Check sheet for the modelled part. Datum: model origin and axes. Units: mm. Face numbers are marked on the shaded views. A direction names the side the tool comes from. Give positions to 0.01 mm unless a question says otherwise; leave off trailing zeros. Write each loop counter-clockwise with the first axis right and the second up, starting at its lowest first coordinate (ties: lowest second). Pieces come first, ordered by that corner, then holes.
from build123d import *

# Parameters (mm, degrees)
SKETCH_1_R      = 1
SKETCH_1_R_2    = 1.5
EXTRUDE_1_DEPTH = 10
SKETCH_3_W      = 58.885714286
SKETCH_3_H      = 63.4
SKETCH_3_W_2    = 54.885714286
SKETCH_3_H_2    = 59.4
EXTRUDE_2_DEPTH = 1.4
FILLET_1_R      = 3


with BuildPart() as part:
    # Эскиз1 → Бобышка-Вытянуть1 (new body)
    with BuildSketch(Plane(origin=(0, 0, 0), x_dir=(1, 0, 0), z_dir=(0, 1, 0))):
        with BuildLine():
            Line((-4, 4), (16, 4))
            ThreePointArc((16, 4), (20, 8), (24, 4))
            Line((24, 4), (62.885714286, 4))
            Line((62.885714286, 4), (62.885714286, 1.233529339))
            ThreePointArc((62.885714286, 1.233529339), (65.2, -2.7), (62.885714286, -6.633529339))
            Line((62.885714286, -6.633529339), (62.885714286, -56.766470661))
            ThreePointArc((62.885714286, -56.766470661), (65.2, -60.7), (62.885714286, -64.633529339))
            Line((62.885714286, -64.633529339), (62.885714286, -67.4))
            Line((62.885714286, -67.4), (24, -67.4))
            ThreePointArc((24, -67.4), (20, -71.4), (16, -67.4))
            Line((16, -67.4), (-4, -67.4))
            Line((-4, -67.4), (-4, -64.866533331))
            ThreePointArc((-4, -64.866533331), (-6.8, -60.7), (-4, -56.533466669))
            Line((-4, -56.533466669), (-4, -6.866533331))
            ThreePointArc((-4, -6.866533331), (-6.8, -2.7), (-4, 1.466533331))
            Line((-4, 1.466533331), (-4, 4))
        make_face()
        with Locations(Location((-2.3, -2.7, 0), (0, 0, 270))):
            Circle(SKETCH_1_R, mode=Mode.SUBTRACT)
        with Locations(Location((60.7, -2.7, 0), (0, 0, 270))):
            Circle(SKETCH_1_R, mode=Mode.SUBTRACT)
        with Locations(Location((60.7, -60.7, 0), (0, 0, 270))):
            Circle(SKETCH_1_R, mode=Mode.SUBTRACT)
        with Locations(Location((-2.3, -60.7, 0), (0, 0, 270))):
            Circle(SKETCH_1_R, mode=Mode.SUBTRACT)
        with Locations(Location((20, -67.4, 0), (0, 0, 270))):
            Circle(SKETCH_1_R_2, mode=Mode.SUBTRACT)
        with Locations(Location((20, 4, 0), (0, 0, 270))):
            Circle(SKETCH_1_R_2, mode=Mode.SUBTRACT)
        with BuildLine():
            Line((1.5, 0), (57.385714286, 0))
            ThreePointArc((57.385714286, 0), (58.446374457, -0.439339828), (58.885714286, -1.5))
            Line((58.885714286, -1.5), (58.885714286, -61.9))
            ThreePointArc((58.885714286, -61.9), (58.446374457, -62.960660172), (57.385714286, -63.4))
            Line((57.385714286, -63.4), (1.5, -63.4))
            ThreePointArc((1.5, -63.4), (0.439339828, -62.960660172), (0, -61.9))
            Line((0, -61.9), (0, -1.5))
            ThreePointArc((0, -1.5), (0.439339828, -0.439339828), (1.5, 0))
        make_face(mode=Mode.SUBTRACT)
    extrude(amount=EXTRUDE_1_DEPTH)

    # Эскиз3 → Бобышка-Вытянуть2 (add)
    with BuildSketch(Plane.XZ):
        with Locations((29.442857143, 31.7)):
            Rectangle(SKETCH_3_W, SKETCH_3_H)
        with Locations((29.442857143, 31.7)):
            Rectangle(SKETCH_3_W_2, SKETCH_3_H_2, mode=Mode.SUBTRACT)
    extrude(amount=-EXTRUDE_2_DEPTH)

    # Скругление1
    # the kernel refuses this fillet: 3 mm, written as the material it takes off along each edge
    with BuildSketch(Plane(origin=(62.885714286, -7.477242159, 67.4), x_dir=(-1, 0, 0), z_dir=(0, 1, 0))) as fillet_1_piece_1:
        with BuildLine():
            CenterArc((2.990896863, -3), FILLET_1_R, 90, 85.535401485)
            Line((0, -2.766470661), (-0.059817937, -2.761800074))
            ThreePointArc((-0.059817937, -2.761800074), (-0.06, -1.38323533), (-0.06, 0))
            Line((-0.06, 0), (0, 0.06))
            Line((0, 0.06), (2.990896863, 0.06))
            Line((2.990896863, 0.06), (2.990896863, 0))
        make_face()
    extrude(amount=24.954484317, mode=Mode.SUBTRACT)
    with BuildSketch(Plane(origin=(-4, -7.408756074, 67.4), x_dir=(0, 0, -1), z_dir=(0, 1, 0))) as fillet_1_piece_2:
        with BuildLine():
            CenterArc((3, -2.96350243), FILLET_1_R, 98.946440174, 81.053559826)
            Line((0, -2.96350243), (-0.06, -2.96350243))
            Line((-0.06, -2.96350243), (-0.06, 0))
            Line((-0.06, 0), (0, 0.06))
            ThreePointArc((0, 0.06), (1.266733334, 0.06), (2.524136002, 0.059270049))
            Line((2.524136002, 0.059270049), (2.533466669, 0))
        make_face()
    extrude(amount=24.817512149, mode=Mode.SUBTRACT)
    with BuildSketch(Plane(origin=(62.885714286, -7.477242159, -4), x_dir=(-1, 0, 0), z_dir=(0, 1, 0))) as fillet_1_piece_3:
        with BuildLine():
            CenterArc((2.990896863, 3), FILLET_1_R, 184.464598515, 85.535401485)
            Line((0, 2.766470661), (-0.059817937, 2.761800074))
            ThreePointArc((-0.059817937, 2.761800074), (-0.06, 1.38323533), (-0.06, 0))
            Line((-0.06, 0), (0, -0.06))
            Line((0, -0.06), (2.990896863, -0.06))
            Line((2.990896863, -0.06), (2.990896863, 0))
        make_face()
    extrude(amount=24.954484317, mode=Mode.SUBTRACT)
    with BuildSketch(Plane(origin=(-4, -7.408756074, -4), x_dir=(0, 0, 1), z_dir=(0, 1, 0))) as fillet_1_piece_4:
        with BuildLine():
            CenterArc((3, 2.96350243), FILLET_1_R, 180, 81.053559826)
            Line((0, 2.96350243), (-0.06, 2.96350243))
            Line((-0.06, 2.96350243), (-0.06, 0))
            Line((-0.06, 0), (0, -0.06))
            ThreePointArc((0, -0.06), (1.266733334, -0.06), (2.524136002, -0.059270049))
            Line((2.524136002, -0.059270049), (2.533466669, 0))
        make_face()
    extrude(amount=24.817512149, mode=Mode.SUBTRACT)


solid = part.part
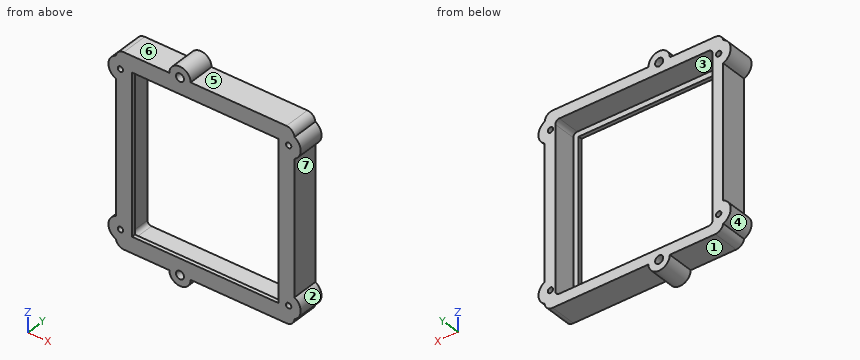
1) Draft check along X on the marked faces 1, 2, 3 and 4. Enter one of: +X half, -X half, draft (parallel to the pull), parting line (faces both ways), or undercut.
2) Sectioned sample at B-B on z = 14.5. Record the boundary of the cut face in (x, y), then the cut area to 3 significant figures.
3) Sectioned sample at A-A on x = 56. Record the boundary of the cut face in (y, z).
4) Sectioned sample at C-C on y = 5.25. Give the number of separate pieces and of enclosed holes in the cut face, then the cut area to 3 significant figures.
5) Scan lines: L1, parallel to X at y = 5, z = 60.7; L2, parallel to Z at x = 35, y = 8; L3, parallel to X at y = 5, z = 20.5. Record each from-to range of solid material in increasing order.
6) Gauge pin test, flat ends, axial feed: pin 1 (5 mm diameter, centred on x = 48, y = 3.5, fed in from +Z); pin 2 (1.5 mm diameter, centred on x = 3.5, y = 2, fed in from -Z); pin 3 (4.5 mm diameter, centred on x = 24, y = 7, fed in from +Z). Record the tip position at first contact, or that the pin passes through.
7) Sectioned sample at D-D on x = 20. Record the boundary of the cut face in (y, z).
8) Access from +Z, -Z, +X, -X, +Y, -Y to the whole of each face (thin tool, end or side, straight path). Record for the marked faces 5, 6 and 7.
Answers below:
1. face 1: draft
1. face 2: +X half
1. face 3: undercut
1. face 4: -X half
2. outline: (-4, 0) - (2, 0) - (2, 1.4) - (0, 1.4) - (0, 10) - (-4, 10) - close; (56.89, 0) - (62.89, 0) - (62.89, 10) - (58.89, 10) - (58.89, 1.4) - (56.89, 1.4) - close
2. area: 85.6 mm2
3. outline: (0, -4) - (10, -4) - (10, 0) - (1.4, 0) - (1.4, 2) - (0, 2) - close; (0, 61.4) - (1.4, 61.4) - (1.4, 63.4) - (10, 63.4) - (10, 67.4) - (0, 67.4) - close
4. separate pieces: 1
4. enclosed holes: 7
4. area: 1,120 mm2
5. L1: x = -6.8 to -3.3, -1.3 to 0, 58.89 to 59.7, 61.7 to 65.2
5. L2: z = -4 to 0, 63.4 to 67.4
5. L3: x = -4 to 0, 58.89 to 62.89
6. pin 1: stops at z = 67.4
6. pin 2: stops at z = -4
6. pin 3: stops at z = 71
7. outline: (0, -8) - (10, -8) - (10, -5.5) - (0, -5.5) - close; (0, -2.5) - (10, -2.5) - (10, 0) - (1.4, 0) - (1.4, 2) - (0, 2) - close; (0, 61.4) - (1.4, 61.4) - (1.4, 63.4) - (10, 63.4) - (10, 65.9) - (0, 65.9) - close; (0, 68.9) - (10, 68.9) - (10, 71.4) - (0, 71.4) - close
8. face 5: +Z, +X, +Y, -Y
8. face 6: +Z, -X, +Y, -Y
8. face 7: +X, +Y, -Y
